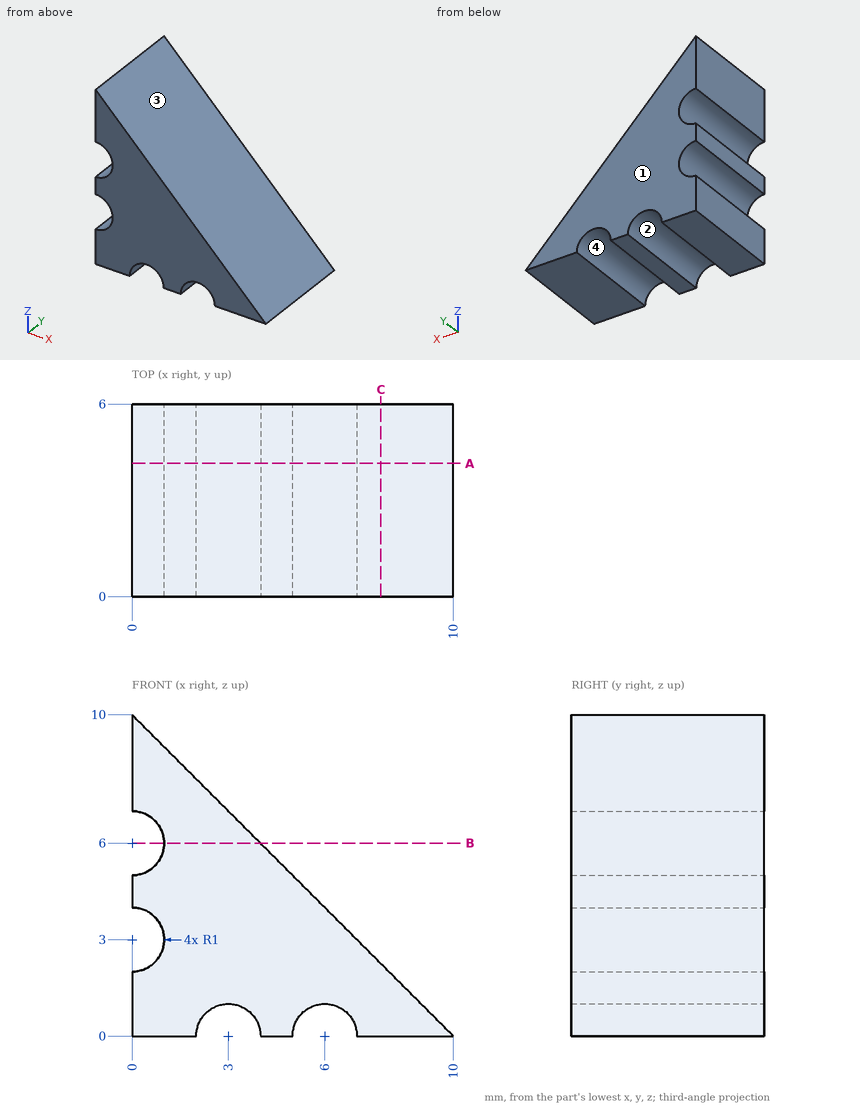
Print and shaded views of the part. All mm, measured from the part's lowest x, y and z. Coordinates: 2 decimals unless noted, no trailing zeros. Order: outer loops, then holes, each group sorted by start corner. A loop starts at its lowest first (then second) coordinate and runs counter-clockwise, first axis right, second up. Notation, with made-up numbers: M 88,62 L 140,62 A21 ccw 140,81 Z; hole C 37.25,64.25 d10. An arc over 180 degrees is marked long. Answer as CSV lines item,"result".
1) Cut at B-B (z = 6). List the corners of the cut face in (x, y).
Verdict:
outline,"M 1,0 L 4,0 L 4,6 L 1,6 Z"
2) Cut at A-A (y = 4.15). List the corners of the cut face in (x, z).
Verdict:
outline,"M 0,0 L 2,0 A1 cw 4,0 L 5,0 A1 cw 7,0 L 10,0 L 0,10 L 0,7 A1 cw 0,5 L 0,4 A1 cw 0,2 Z"
3) Flat gauge pins, fed straight in: P1, Ø3, axis at y = 1, z = 6.5, coming from the +X side; P2, Ø2, axis at x = 7.5, y = 4, coming from the +Z side. Where does each tip first touch, or does it go through?
Verdict:
P1,"x = 5"
P2,"z = 3.5"
4) Mould opens along X. For the marked faces 1, 2, 3 and 4 say: released by +X, released by -X, zero draft, split by the parting line, or undercut.
Verdict:
face 1,"zero draft"
face 2,"undercut"
face 3,"released by +X"
face 4,"undercut"
5) Cut at C-C (x = 7.75). List the corners of the cut face in (y, z), then the cut area to 3 significant figures.
Verdict:
outline,"M 0,0 L 6,0 L 6,2.25 L 0,2.25 Z"
area,"13.5 mm2"
6) Drill centre lines: L1, parallel to X at y = 2.15, z = 0.5; L2, parallel to X at y = 4, z = 0.75. Where is each one in solid material? Low to high. Write a range as from..to.
Verdict:
L1,"0..2.13, 3.87..5.13, 6.87..9.5"
L2,"0..2.34, 3.66..5.34, 6.66..9.25"
